The listing builds one solid part. Answer for the finished solid, in the listing's coordinates (mm). Face numbers are marked on the shaded views. A direction names the side the tool comes from. Give positions to 0.01 mm unless a question says otherwise; leave off trailing zeros. Write each loop counter-clockwise with the first axis right and the second up, starting at its lowest first coordinate (ties: lowest second). Pieces come first, ordered by that corner, then holes. Notation, with made-up numbers: (48, 82.25) -> (102, 82.25) arc R22 ccw to (102, 89.25) -> close; hole circle Ø8 at (23.5, -2.5). An arc over 180 degrees is marked (long way). Write each question's results on one line, items separated by ' | '. Start each with the question number.
from build123d import *

# Parameters (mm, degrees)
SKETCH1_R           = 15
SKETCH1_R_2         = 1.5
SKETCH1_W           = 14
SKETCH1_H           = 12
BOSS_EXTRUDE1_DEPTH = 3


with BuildPart() as part:
    # Sketch1 → Boss-Extrude1 (new body)
    with BuildSketch(Plane.XY):
        Circle(SKETCH1_R)
        with Locations((-12, 0)):
            Circle(SKETCH1_R_2, mode=Mode.SUBTRACT)
        with Locations((12, 0)):
            Circle(SKETCH1_R_2, mode=Mode.SUBTRACT)
        with Locations((0, -4)):
            Rectangle(SKETCH1_W, SKETCH1_H, mode=Mode.SUBTRACT)
    extrude(amount=BOSS_EXTRUDE1_DEPTH)


solid = part.part
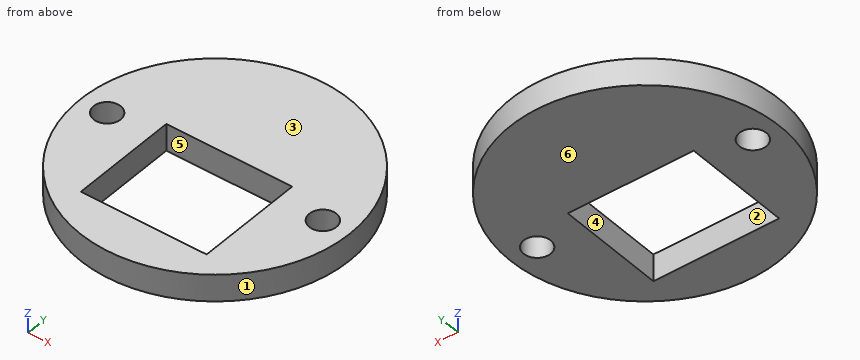
1. Section A-A (x = 0) is taken. Write down the section's boundary in (y, z).
2. Section C-C (z = 1.7) is taken. Write down the section's boundary in (x, y).
3. A tool of negligible diameter and unlimited length cuts with its end or side. For the marked faces 5 and 6, from which of +Z, -Z, +X, -X, +Y, -Y can it reach the whole face along a straight path? Write none if from no direction.
4. Section B-B (y = 0) is taken. Write down the section's boundary in (x, z).
5. The mould has two halves that part along Y. Classify the marked faces 1, 2, 3 and 4: pulls with the +Y half, pulls with the -Y half, needs draft (parallel to the pull), parting line crosses it, or undercut.
6. Each of these flat-tipped pins is pushed along its axis until it touches: pin 1 Ø1.5 at (y, z) = (-5, 1.5) entering from -X; pin 2 Ø1.5 at (y, z) = (-2, 1) entering from +X; pin 3 Ø2.5 at (x, y) = (12, 0) entering from -Z; pin 4 Ø1.5 at (x, z) = (2.5, 0.5) entering from -Y. Where does it stop, or does it pass through?
7. Consider probe 1 along Y at (x, z) = (-4.25, 1.95); probe 2 along Y at (x, z) = (12, 1.1); probe 3 along X at (y, z) = (-9, 1.1). Determine where each line is inside the solid, lowest interval first. Write a range as [from, to].
8. Section D-D (y = -3) is taken. Write down the section's boundary in (x, z).
Results:
1) outline: (-15, 0) -> (-10, 0) -> (-10, 3) -> (-15, 3) -> close; (2, 0) -> (15, 0) -> (15, 3) -> (2, 3) -> close
2) outline: circle Ø30 at (0, 0); hole circle Ø3 at (-12, 0); hole (-7, -10) -> (7, -10) -> (7, 2) -> (-7, 2) -> close; hole circle Ø3 at (12, 0)
3) face 5: +Z, -Z | face 6: -Z, +X, -X, +Y, -Y
4) outline: (-15, 0) -> (-13.5, 0) -> (-13.5, 3) -> (-15, 3) -> close; (-10.5, 0) -> (-7, 0) -> (-7, 3) -> (-10.5, 3) -> close; (7, 0) -> (10.5, 0) -> (10.5, 3) -> (7, 3) -> close; (13.5, 0) -> (15, 0) -> (15, 3) -> (13.5, 3) -> close
5) face 1: parting line crosses it | face 2: undercut | face 3: needs draft | face 4: undercut
6) pin 1: stops at x = -14.39 | pin 2: stops at x = 14.95 | pin 3: passes through | pin 4: stops at y = -14.9
7) probe 1: y = [-14.39, -10], [2, 14.39] | probe 2: y = [-9, -1.5], [1.5, 9] | probe 3: x = [-12, -7], [7, 12]
8) outline: (-14.7, 0) -> (-7, 0) -> (-7, 3) -> (-14.7, 3) -> close; (7, 0) -> (14.7, 0) -> (14.7, 3) -> (7, 3) -> close
